Geometry check sheet. Reference: the model listing, model coordinates, mm. A direction names the side the tool comes from. Give positions to 0.01 mm unless a question says otherwise; leave off trailing zeros. Write each loop counter-clockwise with the first axis right and the second up, starting at its lowest first coordinate (ties: lowest second). Pieces come first, ordered by that corner, then holes. Notation, with made-up numbers: (84.5, 24) - (124.5, 24) arc R8 cw to (124.5, 32) - close; hole circle Ø9 at (17.25, -12). An arc over 180 degrees is marked (long way). Write item = value, one per line. Start each with the question number.
(1) Depth check by flat-ended pin: pin 1 Ø4.5 at (x, z) = (-17, 6) entering from +Y. Enter the tip coordinate at first touch or a pass-through.
(2) Thickness scan on L1, parallel to X at y = -13, z = 7.75; L2, parallel to X at y = 11.7, z = 7.5; L3, parallel to Z at x = 18, y = 0. Record the ranges inside material, lowest first.
(3) Section check A-A, the plane z = 7.5. Enter the section's corners in (x, y).
(4) Access from +Z, -Z, +X, -X, +Y, -Y to the whole of each face (thin tool, end or side, straight path). Record for faces 4 (the cylindrical face through (-18.977, -2.832, 9.856)), 5 (the cylindrical face through (21.794, 12.042, 9.919)).
(5) Section check B-B, the plane y = 0. Enter the section's corners in (x, z), plus the area to 3 significant figures.
(6) Section check D-D, the plane z = 14. Enter the section's corners in (x, y), plus the area to 3 significant figures.
(7) Section check C-C, the plane x = -18. Enter the section's corners in (y, z), plus the area to 3 significant figures.
(8) Draft check along Z on faces 1 (the flat face through (-6, 10, 0)), 2 (the flat face through (0, 15, 7)), 3 (the cylindrical face through (-13.54, 12.04, 6.91)). Enter one of: pulls with the +Z half, pulls with the -Z half, needs draft (parallel to the pull), parting line crosses it, or undercut.
```python
from build123d import *

# Parameters (mm, degrees)
SKETCH_1_W          = 55
SKETCH_1_H          = 30
SKETCH_1_R          = 11
EXTRUDE_1_DEPTH     = 15
SKETCH_2_R          = 2.55
CUT_EXTRUDE_1_DEPTH = 44.373378932
SKETCH_3_R          = 4.5
CUT_EXTRUDE_2_DEPTH = 6
CHAMFER_1_SIZE      = 1


with BuildPart() as part:
    # 草图1 → 凸台-拉伸1 (new body)
    with BuildSketch(Plane.XY):
        Rectangle(SKETCH_1_W, SKETCH_1_H)
        Circle(SKETCH_1_R, mode=Mode.SUBTRACT)
    extrude(amount=EXTRUDE_1_DEPTH)

    # 草图2 → 切除-拉伸1 (cut, through all)
    with BuildSketch(Plane(origin=(0, 15, 0), x_dir=(1, 0, 0), z_dir=(0, 1, 0))):
        with Locations(Location((-18, -7.5, 0), (0, 0, 270))):
            Circle(SKETCH_2_R)
        with Locations(Location((18, -7.5, 0), (0, 0, 90))):
            Circle(SKETCH_2_R)
    extrude(amount=-CUT_EXTRUDE_1_DEPTH, mode=Mode.SUBTRACT)

    # 草图3 → 切除-拉伸2 (cut)
    with BuildSketch(Plane(origin=(0, 15, 0), x_dir=(1, 0, 0), z_dir=(0, 1, 0))):
        with Locations(Location((-18, -7.5, 0), (0, 0, 270))):
            Circle(SKETCH_3_R)
        with Locations(Location((18, -7.5, 0), (0, 0, 270))):
            Circle(SKETCH_3_R)
    extrude(amount=-CUT_EXTRUDE_2_DEPTH, mode=Mode.SUBTRACT)

    # 倒角1
    chamfer_1_edges = [part.edges().sort_by_distance(p)[0] for p in [
        (-27.5, 15, 7.5),
        (27.5, 15, 7.5),
        (27.5, -15, 7.5),
        (-27.5, -15, 7.5),
    ]]
    chamfer(chamfer_1_edges, length=CHAMFER_1_SIZE)


solid = part.part
```
Model answer:
q1.pin_1 = 9
q2.L1 = -27.5 to -20.54, -15.46 to 15.46, 20.54 to 27.5
q2.L2 = -27.5 to -22.5, -13.5 to 13.5, 22.5 to 27.5
q2.L3 = 0 to 4.95, 10.05 to 15
q3.outline = (-27.5, -14) - (-26.5, -15) - (-20.55, -15) - (-20.55, 9) - (-22.5, 9) - (-22.5, 15) - (-26.5, 15) - (-27.5, 14) - close; (-15.45, -15) - (15.45, -15) - (15.45, 9) - (13.5, 9) - (13.5, 15) - (-13.5, 15) - (-13.5, 9) - (-15.45, 9) - close; (20.55, -15) - (26.5, -15) - (27.5, -14) - (27.5, 14) - (26.5, 15) - (22.5, 15) - (22.5, 9) - (20.55, 9) - close; hole circle Ø22 at (0, 0)
q4.face_4 = +Y, -Y
q4.face_5 = +Y
q5.outline = (-27.5, 0) - (-11, 0) - (-11, 15) - (-27.5, 15) - close; (11, 0) - (27.5, 0) - (27.5, 15) - (11, 15) - close; hole circle Ø5.1 at (-18, 7.5); hole circle Ø5.1 at (18, 7.5)
q5.area = 454 mm²
q6.outline = (-27.5, -14) - (-26.5, -15) - (26.5, -15) - (27.5, -14) - (27.5, 14) - (26.5, 15) - (-26.5, 15) - (-27.5, 14) - close; hole circle Ø22 at (0, 0)
q6.area = 1,270 mm²
q7.outline = (-15, 0) - (15, 0) - (15, 3) - (9, 3) - (9, 4.95) - (-15, 4.95) - close; (-15, 10.05) - (9, 10.05) - (9, 12) - (15, 12) - (15, 15) - (-15, 15) - close
q7.area = 274 mm²
q8.face_1 = pulls with the -Z half
q8.face_2 = needs draft
q8.face_3 = undercut
